from build123d import *

# Parameters (mm, degrees)
F0_W     = 304.8
F0_H     = 304.8
F1_DEPTH = 12.7
F2_D     = 7.9375
F2_DEPTH = 20.6629
F2_TIP   = 2.3846655818
F3_D     = 16.66748
F3_DEPTH = 20.6756
F3_TIP   = 5.0074161752


with BuildPart() as f1:
    # F0 (on Top) → F1 (new body)
    with BuildSketch(Plane.XY):
        with Locations((-152.4, 152.4)):
            Rectangle(F0_W, F0_H)
    extrude(amount=-F1_DEPTH)

    # F2
    with Locations(Plane.XY):
        with Locations((-263.525, 279.4), (-263.525, 152.4), (-263.525, 25.4), (-41.275, 279.4), (-41.275, 152.4), (-41.275, 25.4)):
            Hole(F2_D / 2, depth=F2_DEPTH)
            with Locations((0, 0, -(F2_DEPTH + F2_TIP / 2))):  # 118° drill point
                Cone(0, F2_D / 2, F2_TIP, mode=Mode.SUBTRACT)

    # F3
    with Locations(Plane.XY):
        with Locations((-215.9, 280.9875), (-88.9, 280.9875), (-88.9, 96.8375), (-215.9, 96.8375)):
            Hole(F3_D / 2, depth=F3_DEPTH)
            with Locations((0, 0, -(F3_DEPTH + F3_TIP / 2))):  # 118° drill point
                Cone(0, F3_D / 2, F3_TIP, mode=Mode.SUBTRACT)


solid = f1.part
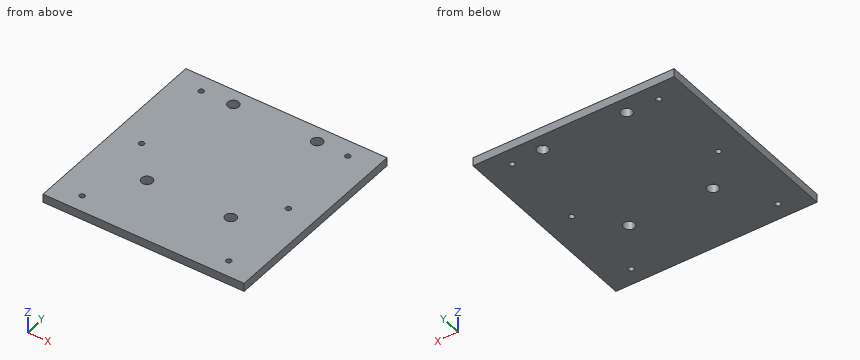
Geometry: final body of the model. Coordinates: model frame, mm. Give positions to 0.01 mm unless a question says otherwise; leave off trailing zeros. Write each loop counter-clockwise with the first axis right and the second up, starting at its lowest first coordinate (ties: lowest second). Pieces come first, ordered by that corner, then holes. Notation, with made-up numbers: M -30.75,27 L -6.75,27 A3 ccw -6.75,31 Z; hole C 57,-16 d8. An arc over 180 degrees is marked long. Answer in a Markdown table with one row per item. Add a question column.
(1) Section B-B on x = -215.9. Return loops of the section in (y, z).
(2) Section A-A on y = 152.4. Return loops of the section in (x, z), and give its area (3 significant figures).
(3) Ray query, line 1 (Y direction, x = -88.9, z = -3.75); line 2 (Y direction, x = -39.5, z = -11.75); line 3 (X direction, y = 279.4, z = -8.5). Return the intervals inside material, ascending.
Result set:
| question | item | result |
|---|---|---|
| 1 | outline | M 0,-12.7 L 88.5,-12.7 L 88.5,0 L 0,0 Z; M 105.17,-12.7 L 272.65,-12.7 L 272.65,0 L 105.17,0 Z; M 289.32,-12.7 L 304.8,-12.7 L 304.8,0 L 289.32,0 Z |
| 2 | outline | M -304.8,-12.7 L -267.49,-12.7 L -267.49,0 L -304.8,0 Z; M -259.56,-12.7 L -45.24,-12.7 L -45.24,0 L -259.56,0 Z; M -37.31,-12.7 L 0,-12.7 L 0,0 L -37.31,0 Z |
| 2 | area | 3,670 mm^2 |
| 3 | line 1 | y = 0 to 88.5, 105.17 to 272.65, 289.32 to 304.8 |
| 3 | line 2 | y = 0 to 21.85, 28.95 to 148.85, 155.95 to 275.85, 282.95 to 304.8 |
| 3 | line 3 | x = -304.8 to -267.49, -259.56 to -224.08, -207.72 to -97.08, -80.72 to -45.24, -37.31 to 0 |
